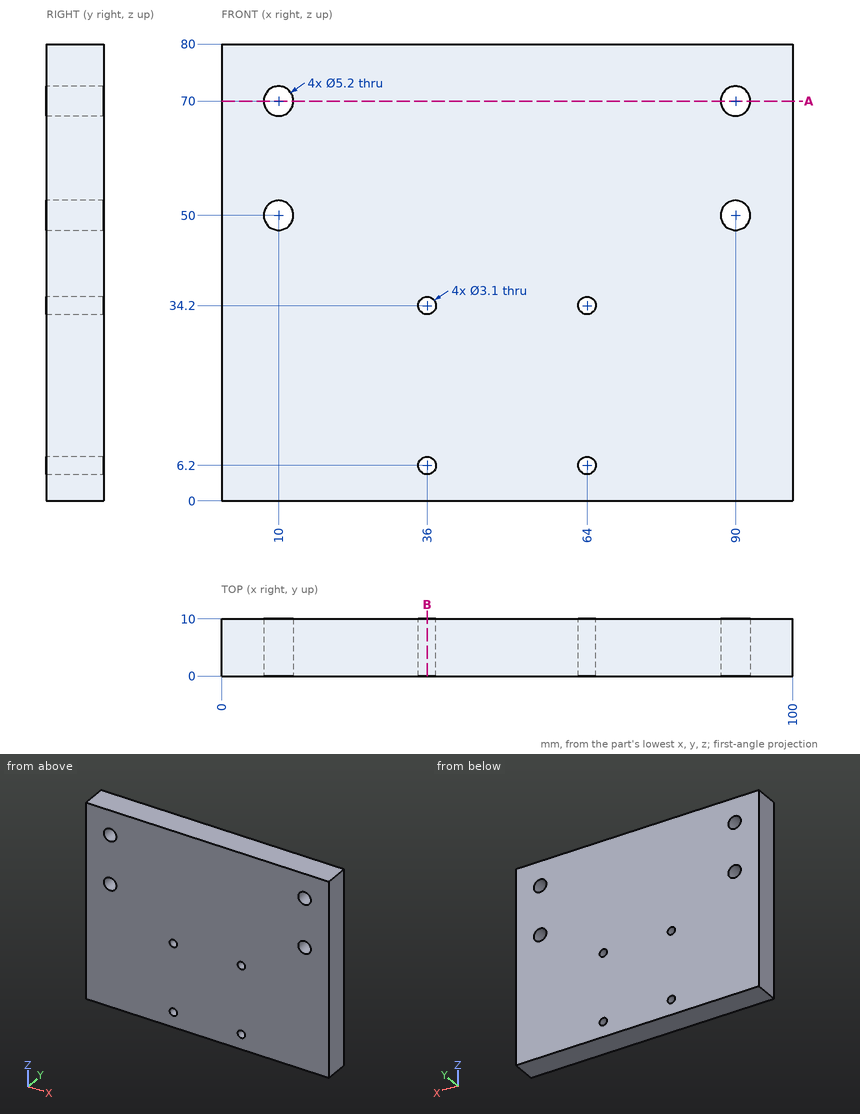
Could you check a few things on this drawing? It's one solid part, dimensions in mm from its lowest x, y, z. Give positions to 0.01 mm unless a question says otherwise; leave off trailing zeros. Order: outer loops, then holes, each group sorted by start corner. A loop starts at its lowest first (then second) coordinate and runs counter-clockwise, first axis right, second up. Notation, with made-up numbers: M -17.5,-9.75 L 38.5,-9.75 A7 cw 38.5,-1.75 Z; hole C 33.5,62 d8. An arc over 180 degrees is marked long. Use one line per item in the form item = value. Start each with the question number.
Item 1: If we section it at B-B (x = 36): Write out the boundary of the cut face in (y, z).
Item 2: If we section it at A-A (z = 70): Write out the boundary of the cut face in (x, y).
Item 3: Will this pin go through, and if not, where does the flat tip stop? pin 1 Ø4.5 at (x, z) = (90, 50) entering from +Y.
Item 4: If I drill on line 1 along X through (y, z) = (4.75, 6.2); line 2 along Z through (x, y) = (90, 1.25); line 3 along Z through (x, y) = (64, 6.25), over which ranges is the centre line in solid material (lowest first)?
Outcome:
q1.outline = M 0,0 L 10,0 L 10,4.65 L 0,4.65 Z; M 0,7.75 L 10,7.75 L 10,32.65 L 0,32.65 Z; M 0,35.75 L 10,35.75 L 10,80 L 0,80 Z
q2.outline = M 0,0 L 7.4,0 L 7.4,10 L 0,10 Z; M 12.6,0 L 87.4,0 L 87.4,10 L 12.6,10 Z; M 92.6,0 L 100,0 L 100,10 L 92.6,10 Z
q3.pin_1 = through
q4.line_1 = 0 to 34.45, 37.55 to 62.45, 65.55 to 100
q4.line_2 = 0 to 47.4, 52.6 to 67.4, 72.6 to 80
q4.line_3 = 0 to 4.65, 7.75 to 32.65, 35.75 to 80
